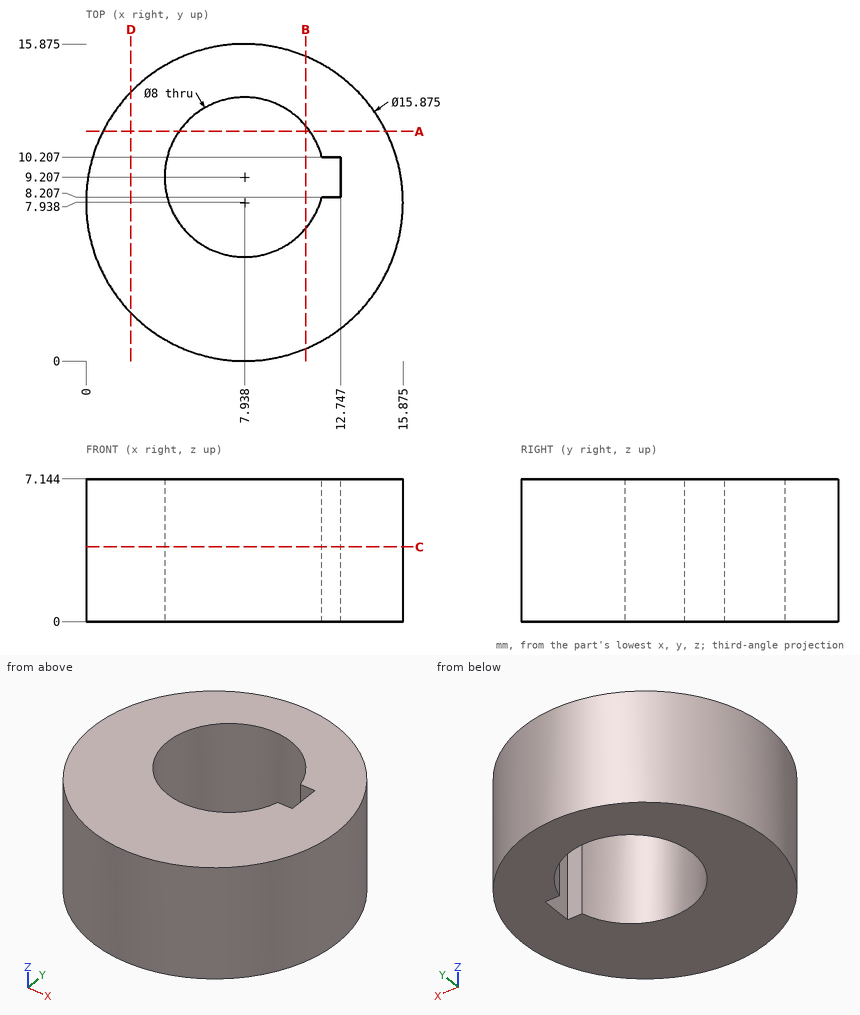
Verification items for this drawing (mm, ordinates from the low corner). Round coordinates to 2 decimals unless told otherwise and drop trailing zeros. Write each loop counter-clockwise with the first axis right and the second up, starting at its lowest first coordinate (ties: lowest second). Pieces come first, ordered by that corner, then holes. Notation, with made-up numbers: (-14.5, -3.5) - (41.5, -3.5) arc R25 cw to (41.5, 32.5) - close; hole circle Ø4 at (70.5, -1). An arc over 180 degrees is marked (long way). Answer as a JSON object with one key per item and string values. Group by question number.
Q1. Section check B-B, the plane x = 11. Enter the section's corners in (y, z) (1 decimal).
Q2. Section check D-D, the plane x = 2.25. Enter the section's corners in (y, z) (1 decimal), plus the area to 3 significant figures.
Q3. Go/stop test with flat-tipped pins: pin 1 Ø1.6 at (y, z) = (9, 3.5) entering from -X; pin 2 Ø4 at (x, z) = (2.5, 5) entering from +Y; pin 3 Ø6.5 at (x, y) = (7.94, 9.21) entering from -Z; pin 4 Ø3 at (x, z) = (12.5, 6.5) entering from -Y (1 decimal). Record where each tip stops, or that it passes through.
Q4. Section check C-C, the plane z = 3.75. Enter the section's corners in (x, y) (1 decimal).
Q5. Thickness scan on line 1 (Y direction, x = 8, z = 1.75) (1 decimal); line 2 (Y direction, x = 11.5, z = 3.25) (1 decimal); line 3 (X direction, y = 7, z = 3.75) (1 decimal). Record the ranges inside material, lowest first.
Q6. Section check A-A, the plane y = 11.5. Enter the section's corners in (x, z) (1 decimal).
Found:
{
 "1": {"outline": "(0.6, 0) - (6.6, 0) - (6.6, 7.1) - (0.6, 7.1) - close; (11.8, 0) - (15.3, 0) - (15.3, 7.1) - (11.8, 7.1) - close"},
 "2": {"outline": "(2.4, 0) - (13.5, 0) - (13.5, 7.1) - (2.4, 7.1) - close", "area": "79.1 mm^2"},
 "3": {"pin 1": "stops at x = 0", "pin 2": "stops at y = 15.09", "pin 3": "passes through", "pin 4": "stops at y = 0.6"},
 "4": {"outline": "circle Ø15.9 at (7.9, 7.9); hole (11.8, 8.2) - (12.7, 8.2) - (12.7, 10.2) - (11.8, 10.2) arc R4 ccw (long way) to start"},
 "5": {"line 1": "y = 0 to 5.2, 13.2 to 15.9", "line 2": "y = 0.8 to 7.4, 11 to 15", "line 3": "x = 0.1 to 4.6, 11.3 to 15.8"},
 "6": {"outline": "(0.8, 0) - (4.7, 0) - (4.7, 7.1) - (0.8, 7.1) - close; (11.2, 0) - (15, 0) - (15, 7.1) - (11.2, 7.1) - close"}
}
